For this review, take the finished solid that the model builds, in its own axes (mm). Coordinates: 2 decimals unless noted, no trailing zeros. Write each loop counter-clockwise with the first axis right and the second up, starting at its lowest first coordinate (ties: lowest second). Pieces come first, ordered by that corner, then holes. Notation, with made-up numbers: (85, 81.25) - (138, 81.25) arc R24 ccw to (138, 105.25) - close; hole circle Ø9 at (-9, 80). An arc over 180 degrees is marked (long way). Write each question's results on one line, items separated by ' | '.
from build123d import *

# Parameters (mm, degrees)
SKETCH1_R           = 4.3
BOSS_EXTRUDE1_DEPTH = 10


with BuildPart() as part:
    # Sketch1 → Boss-Extrude1 (new body)
    with BuildSketch(Plane.XY):
        with BuildLine():
            Line((-8.786321272, 52.647017374), (-17.697634828, 56.188182479))
            add(Edge.make_bspline(
                [(-35.179619379, 30.460455257), (-35.223518874, 33.917669849), (-34.201169153, 49.781165774), (-23.152962073, 54.671871571), (-17.697634828, 56.188182479)],
                knots=[0, 0, 0, 0, 0.555505608, 1, 1, 1, 1], degree=3))
            ThreePointArc((-35.179619379, 30.460455257), (-26.179619379, 21.460455257), (-17.179619379, 30.460455257))
            add(Edge.make_bspline(
                [(-17.179619379, 30.460455257), (-17.07332671, 33.217532109), (-22.036687674, 41.830328863), (-16.393122833, 53.508799667), (-8.786321272, 52.647017374)],
                knots=[0, 0, 0, 0, 0.305227292, 1, 1, 1, 1], degree=3))
        make_face()
        with Locations((-26.179619379, 30.460455257)):
            Circle(SKETCH1_R, mode=Mode.SUBTRACT)
    extrude(amount=BOSS_EXTRUDE1_DEPTH)


solid = part.part
Q1. Mouldability with a two-part tool opening along Y and no side actions: class faces 1 (the face through (-26.378, 21.463, 4.93)), 2 (the face through (-13.2, 54.4, 4.9)), 3 (the face through (-26.739, 34.724, 4.93)) as pulls with the +Y half, pulls with the -Y half, needs draft (parallel to the pull), parting line crosses it, or undercut.
Results found:
face 1: pulls with the -Y half | face 2: pulls with the +Y half | face 3: undercut
Q2. Wall thickness on line 1 along X through (y, z) = (33.5, 7.25); line 2 along Y through (x, z) = (-25.5, 2.75); line 3 along X through (y, z) = (29.5, 7.5): over which ranges is each line inside the solid? List them lowest first. Write a range as from..to.
Results found:
line 1: -35.09..-29.22, -23.14..-17.6 | line 2: 21.49..26.21, 34.71..53.11 | line 3: -35.13..-30.37, -21.99..-17.23
Q3. Take a section at A-A on y = 24.5. State the section outline as (x, z) points, plus the area to 3 significant figures.
Results found:
outline: (-32.92, 0) - (-19.44, 0) - (-19.44, 10) - (-32.92, 10) - close | area: 135 mm2
Q4. For pin 1 (1 mm diameter, centred on x = -23.5, z = 6.5, fed in from -Y); pin 2 (1 mm diameter, centred on y = 49, z = 5.5, fed in from -X); pin 3 (5 mm diameter, centred on x = -13, z = 3, fed in from +Y); pin 4 (5 mm diameter, centred on x = -26.18, y = 30.46, fed in from -Z), all flat-tipped, find the tip position at first contact; note any pin that passes through.
Results found:
pin 1: y = 21.73 | pin 2: x = -30.75 | pin 3: y = 55.31 | pin 4: through
